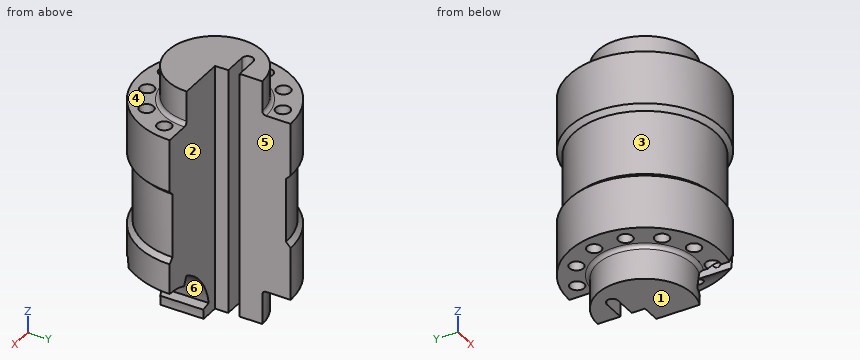
from build123d import *

# Parameters (mm, degrees)
CUT_EXTRUDE1_DEPTH      = 66.5
CUT_EXTRUDE1_DEPTH_BACK = 66.5
CUT_EXTRUDE3_DEPTH      = 41
SKETCH4_R               = 3.75
CUT_EXTRUDE4_DEPTH      = 66.5000001
CUT_EXTRUDE4_DEPTH_BACK = 66.5000001


with BuildPart() as part:
    # Sketch1 → Revolve1 (revolve)
    with BuildSketch(Plane(origin=(0, 0, 0), x_dir=(0, 0, -1), z_dir=(1, 0, 0))):
        with BuildLine():
            Line((65.5, 0), (-65.5, 0))
            Line((-65.5, 0), (-65.5, 25))
            Line((-65.5, 25), (-49.5, 25))
            ThreePointArc((-49.5, 25), (-48.085786438, 25.585786438), (-47.5, 27))
            Line((-47.5, 27), (-47.5, 40))
            Line((-47.5, 40), (-19.5, 40))
            Line((-19.5, 40), (-17, 37.5))
            Line((-17, 37.5), (17, 37.5))
            Line((17, 37.5), (19.5, 40))
            Line((19.5, 40), (47.5, 40))
            Line((47.5, 40), (47.5, 27))
            ThreePointArc((47.5, 27), (48.085786438, 25.585786438), (49.5, 25))
            Line((49.5, 25), (65.5, 25))
            Line((65.5, 25), (65.5, 0))
        make_face()
    revolve(axis=Axis((0, 0, -65.5), (0, 0, 1)))

    # Sketch2 → Cut-Extrude1 (cut, two sides)
    with BuildSketch(Plane.XY) as cut_extrude1_sk:
        with BuildLine():
            Line((0, 40), (0, 13))
            Line((0, 13), (-12, 13))
            ThreePointArc((-12, 13), (-15, 10), (-12, 7))
            Line((-12, 7), (0, 7))
            Line((0, 7), (0, 0))
            Line((0, 0), (40, 0))
            ThreePointArc((40, 0), (28.284271247, 28.284271247), (0, 40))
        make_face()
    extrude(amount=CUT_EXTRUDE1_DEPTH, mode=Mode.SUBTRACT)
    extrude(cut_extrude1_sk.sketch, amount=-CUT_EXTRUDE1_DEPTH_BACK, mode=Mode.SUBTRACT)

    # Sketch3 → Cut-Extrude3 (cut, through all)
    with BuildSketch(Plane(origin=(0, 0, 0), x_dir=(1, 0, 0), z_dir=(0, 1, 0))):
        with BuildLine():
            Line((27.321452148, 38.310766389), (25.208360839, 33.779227454))
            ThreePointArc((25.208360839, 33.779227454), (12.23263309, 44.193349985), (5.531728645, 59.422313782))
            Line((5.531728645, 59.422313782), (10.45576741, 60.29055467))
            ThreePointArc((10.45576741, 60.29055467), (63.800600209, 83.76284287), (27.321452148, 38.310766389))
        make_face()
    extrude(amount=-CUT_EXTRUDE3_DEPTH, mode=Mode.SUBTRACT)

    # Sketch4 → Cut-Extrude4 (cut, two sides)
    with BuildSketch(Plane.XY) as cut_extrude4_sk:
        with Locations((-8.282209443, 30.909626441)):
            Circle(SKETCH4_R)
        with Locations((8.282209443, 30.909626441)):
            Circle(SKETCH4_R)
        with Locations((22.627416998, 22.627416998)):
            Circle(SKETCH4_R)
        with Locations((30.909626441, 8.282209443)):
            Circle(SKETCH4_R)
        with Locations((30.909626441, -8.282209443)):
            Circle(SKETCH4_R)
        with Locations((22.627416998, -22.627416998)):
            Circle(SKETCH4_R)
        with Locations((8.282209443, -30.909626441)):
            Circle(SKETCH4_R)
        with Locations((-8.282209443, -30.909626441)):
            Circle(SKETCH4_R)
        with Locations((-22.627416998, -22.627416998)):
            Circle(SKETCH4_R)
        with Locations((-30.909626441, -8.282209443)):
            Circle(SKETCH4_R)
        with Locations((-30.909626441, 8.282209443)):
            Circle(SKETCH4_R)
        with Locations((-22.627416998, 22.627416998)):
            Circle(SKETCH4_R)
    extrude(amount=CUT_EXTRUDE4_DEPTH, mode=Mode.SUBTRACT)
    extrude(cut_extrude4_sk.sketch, amount=-CUT_EXTRUDE4_DEPTH_BACK, mode=Mode.SUBTRACT)


solid = part.part
Build history of the part. All positions in model axes, mm. Face numbers are marked on the shaded views. A direction names the side the tool comes from. Coordinates: 2 decimals unless noted, no trailing zeros. Write each loop counter-clockwise with the first axis right and the second up, starting at its lowest first coordinate (ties: lowest second). Pieces come first, ordered by that corner, then holes.
(1) Cut at A-A on z = 54. List the corners of the cut face in (x, y).
(2) Pin check, flat tips, straight feed: pin 1 Ø12 at (y, z) = (-21.5, -28.5) entering from -X; pin 2 Ø12 at (x, y) = (-22.63, 22.63) entering from +Z; pin 3 Ø5 at (y, z) = (-4, 36.5) entering from +X. Stop position of each tip, or through.
(3) Drill centre lines: line 1 (X direction, y = -19.5, z = -9); line 2 (X direction, y = -6, z = 26); line 3 (Y direction, x = -11.5, z = -15). Where is each one in solid material? Low to high.
(4) Mould opens along Z. For the marked faces 1, 2 and 3 say: pulls with the +Z half, pulls with the -Z half, needs draft (parallel to the pull), parting line crosses it, or undercut.
(5) Cut at B-B on z = 34. State how many separate pieces and enclosed holes the cut face has, and give its area (3 significant figures).
(6) 3-axis set-ups, long thin cutter, end or side, ignore diameter. For the marked faces 4, 5 and 6: which of +Z, -Z, +X, -X, +Y, -Y reach the whole face in a straight line?
Working result:
1. outline: (-12, 7) arc R3 cw to (-12, 13) - (0, 13) - (0, 25) arc R25 ccw (long way) to (25, 0) - (0, 0) - (0, 7) - close
2. pin 1: stops at x = -36.87
2. pin 2: stops at z = 47.77
2. pin 3: stops at x = 39.97
3. line 1: x = -32.03 to -24.7, -20.56 to 20.56, 24.7 to 32.03
3. line 2: x = -39.55 to -33.89, -27.93 to 27.93, 33.89 to 39.55
3. line 3: y = -35.69 to -32.84, -28.98 to 7, 13 to 28.98, 32.84 to 35.69
4. face 1: pulls with the -Z half
4. face 2: needs draft
4. face 3: undercut
5. separate pieces: 1
5. enclosed holes: 9
5. area: 3,290 mm2
6. face 4: +Z
6. face 5: +Z, -Z, +X, +Y
6. face 6: +Y, -Y
